from build123d import *

# Parameters (mm, degrees)
SKETCH1_R           = 1.5
SKETCH1_R_2         = 55
BOSS_EXTRUDE1_DEPTH = 3.175
CUT_EXTRUDE3_DEPTH  = 140.736059076
CUT_EXTRUDE4_START  = -10
SKETCH3_R           = 1.5
CUT_EXTRUDE4_DEPTH  = 10
CUT_EXTRUDE5_DEPTH  = 140.736059076
CUT_EXTRUDE6_DEPTH  = 140.736059076
SKETCH6_R           = 1.5
CUT_EXTRUDE7_DEPTH  = 124.953233311
SKETCH7_W           = 69.762043991
SKETCH7_H           = 61.208981149
CUT_EXTRUDE8_DEPTH  = 100


with BuildPart() as part:
    # Sketch1 → Boss-Extrude1 (new body)
    with BuildSketch(Plane(origin=(0, 0, 0), x_dir=(1, 0, 0), z_dir=(0, 1, 0))):
        Polygon((0.047005036, -98.782806148), (-98.782806148, -0.047005036), (-0.047005036, 98.782806148), (98.782806148, 0.047005036), align=None)
        with Locations(Location((-61.346730494, 5.55625, 0), (0, 0, 270))):
            Circle(SKETCH1_R, mode=Mode.SUBTRACT)
        with Locations(Location((-61.346730494, -5.55625, 0), (0, 0, 270))):
            Circle(SKETCH1_R, mode=Mode.SUBTRACT)
        with Locations(Location((-5.55625, -61.346730494, 0), (0, 0, 270))):
            Circle(SKETCH1_R, mode=Mode.SUBTRACT)
        with Locations(Location((5.55625, -61.346730494, 0), (0, 0, 270))):
            Circle(SKETCH1_R, mode=Mode.SUBTRACT)
        with Locations(Location((61.346730494, -5.55625, 0), (0, 0, 270))):
            Circle(SKETCH1_R, mode=Mode.SUBTRACT)
        with Locations(Location((61.346730494, 5.55625, 0), (0, 0, 270))):
            Circle(SKETCH1_R, mode=Mode.SUBTRACT)
        with Locations(Location((5.55625, 61.346730494, 0), (0, 0, 270))):
            Circle(SKETCH1_R, mode=Mode.SUBTRACT)
        with Locations(Location((-5.55625, 61.346730494, 0), (0, 0, 270))):
            Circle(SKETCH1_R, mode=Mode.SUBTRACT)
        with Locations(Location((0, 0, 0), (0, 0, 270))):
            Circle(SKETCH1_R_2, mode=Mode.SUBTRACT)
    extrude(amount=BOSS_EXTRUDE1_DEPTH)

    # Sketch2 → Cut-Extrude3 (cut, through all)
    with BuildSketch(Plane(origin=(0, 3.175, 0), x_dir=(1, 0, 0), z_dir=(0, 1, 0))):
        Polygon((3.175, 53.34), (3.175, 59.69), (-3.175, 59.69), (-3.175, 53.34), (-3.175, 52.244537665), (3.175, 52.244537665), align=None)
        Polygon((53.34, -3.175), (59.69, -3.175), (59.69, 3.175), (53.34, 3.175), (52.244537665, 3.175), (52.244537665, -3.175), align=None)
        Polygon((-3.175, -53.34), (-3.175, -59.69), (3.175, -59.69), (3.175, -53.34), (3.175, -52.244537665), (-3.175, -52.244537665), align=None)
        Polygon((-53.34, 3.175), (-59.69, 3.175), (-59.69, -3.175), (-53.34, -3.175), (-52.244537665, -3.175), (-52.244537665, 3.175), align=None)
    extrude(amount=-CUT_EXTRUDE3_DEPTH, mode=Mode.SUBTRACT)

    # Sketch3 → Cut-Extrude4 (cut)
    # profile 1 of 3: a face of its own
    with BuildSketch(Plane(origin=(0, 3.175, 0), x_dir=(1, 0, 0), z_dir=(0, 1, 0)).offset(CUT_EXTRUDE4_START)):
        with BuildLine():
            Line((38.872362643, 38.909374482), (49.367900556, 49.414905592))
            Line((49.367900556, 49.414905592), (24.66044776, 74.09885587))
            Line((24.66044776, 74.09885587), (5.321919094, 54.741914263))
            ThreePointArc((5.321919094, 54.741914263), (23.472344653, 49.739813394), (38.872362643, 38.909374482))
        make_face()
    # profile 2 of 3: a face of its own
    with BuildSketch(Plane(origin=(0, 3.175, 0), x_dir=(1, 0, 0), z_dir=(0, 1, 0)).offset(CUT_EXTRUDE4_START)):
        with BuildLine():
            Line((-49.367900556, -49.414905592), (-38.872362643, -38.909374482))
            ThreePointArc((-38.872362643, -38.909374482), (-49.717452606, -23.519670626), (-54.736824686, -5.374013707))
            Line((-54.736824686, -5.374013707), (-74.075353352, -24.730955314))
            Line((-74.075353352, -24.730955314), (-49.367900556, -49.414905592))
        make_face()
    # profile 3 of 3: a face of its own
    with BuildSketch(Plane(origin=(0, 3.175, 0), x_dir=(1, 0, 0), z_dir=(0, 1, 0)).offset(CUT_EXTRUDE4_START)):
        with BuildLine():
            Line((98.782806148, 0.047005036), (49.367900556, 49.414905592))
            Line((49.367900556, 49.414905592), (38.872362643, 38.909374482))
            ThreePointArc((38.872362643, 38.909374482), (50.179066182, 22.518022052), (54.908281479, 3.175))
            Line((54.908281479, 3.175), (59.69, 3.175))
            Line((59.69, 3.175), (59.69, -3.175))
            Line((59.69, -3.175), (54.908281479, -3.175))
            ThreePointArc((54.908281479, -3.175), (38.890872965, -38.890872965), (3.175, -54.908281479))
            Line((3.175, -54.908281479), (3.175, -59.69))
            Line((3.175, -59.69), (-3.175, -59.69))
            Line((-3.175, -59.69), (-3.175, -54.908281479))
            ThreePointArc((-3.175, -54.908281479), (-22.494142184, -50.189775527), (-38.872362643, -38.909374482))
            Line((-38.872362643, -38.909374482), (-49.367900556, -49.414905592))
            Line((-49.367900556, -49.414905592), (0.047005036, -98.782806148))
            Line((0.047005036, -98.782806148), (98.782806148, 0.047005036))
        make_face()
        with Locations((-5.55625, -61.346730494)):
            Circle(SKETCH3_R, mode=Mode.SUBTRACT)
        with Locations((5.55625, -61.346730494)):
            Circle(SKETCH3_R, mode=Mode.SUBTRACT)
        with Locations((61.346730494, -5.55625)):
            Circle(SKETCH3_R, mode=Mode.SUBTRACT)
        with Locations((61.346730494, 5.55625)):
            Circle(SKETCH3_R, mode=Mode.SUBTRACT)
    extrude(amount=CUT_EXTRUDE4_DEPTH, mode=Mode.SUBTRACT)

    # Sketch4 → Cut-Extrude5 (cut, through all)
    with BuildSketch(Plane(origin=(0, 3.175, 0), x_dir=(1, 0, 0), z_dir=(0, 1, 0))):
        Polygon((-54.908281479, 3.175), (-75.255419375, 23.502783048), (-23.546766486, 75.260669691), (-3.175, 54.908281479), align=None)
    extrude(amount=-CUT_EXTRUDE5_DEPTH, mode=Mode.SUBTRACT)


with BuildPart() as cut_extrude5_piece_1:
    # of the separate pieces the step leaves, piece 1, a body of its own (cut_extrude5_pieces)
    add(part.part.solids().sort_by_distance((-74.075353352, 0, 24.730955314))[0])


with BuildPart() as cut_extrude5_piece_2:
    # of the separate pieces the step leaves, piece 2, a body of its own (cut_extrude5_pieces)
    add(part.part.solids().sort_by_distance((-3.175, 0, -54.908281479))[0])


with BuildPart() as cut_extrude6_tool:
    # Sketch5 → Cut-Extrude6 (new, through all)
    with BuildSketch(Plane(origin=(0, 3.175, 0), x_dir=(1, 0, 0), z_dir=(0, 1, 0))):
        Polygon((-0.047005036, 98.782806148), (11.121699276, 87.624725864), (-87.614101836, -11.205085321), (-98.782806148, -0.047005036), align=None)
    extrude(amount=-CUT_EXTRUDE6_DEPTH)


with BuildPart() as cut_extrude5_piece_1_1:
    add(cut_extrude5_piece_1.part)

    # Cut-Extrude6: cut by cut_extrude6_tool
    add(cut_extrude6_tool.part, mode=Mode.SUBTRACT)


with BuildPart() as cut_extrude5_piece_2_1:
    add(cut_extrude5_piece_2.part)

    # Cut-Extrude6: cut by cut_extrude6_tool
    add(cut_extrude6_tool.part, mode=Mode.SUBTRACT)


with BuildPart() as cut_extrude7_tool:
    # Sketch6 → Cut-Extrude7 (new, through all)
    with BuildSketch(Plane(origin=(0, 3.175, 0), x_dir=(1, 0, 0), z_dir=(0, 1, 0))):
        with BuildLine():
            ThreePointArc((-73.220428508, -14.983508678), (-73.219419094, -17.104828781), (-71.09809899, -17.103819368))
            Line((-71.09809899, -17.103819368), (-73.220428508, -14.983508678))
        make_face()
        with BuildLine():
            Line((-73.220428508, -14.983508678), (-71.09809899, -17.103819368))
            ThreePointArc((-71.09809899, -17.103819368), (-70.773307917, -16.617359439), (-70.659263749, -16.043664023))
            ThreePointArc((-70.659263749, -16.043664023), (-71.585568332, -14.657708191), (-73.220428508, -14.983508678))
        make_face()
        with BuildLine():
            ThreePointArc((-79.989802749, -8.220573681), (-79.988793336, -10.341893785), (-77.867473232, -10.340884371))
            Line((-77.867473232, -10.340884371), (-79.989802749, -8.220573681))
        make_face()
        with BuildLine():
            Line((-79.989802749, -8.220573681), (-77.867473232, -10.340884371))
            ThreePointArc((-77.867473232, -10.340884371), (-77.542682159, -9.854424443), (-77.428637991, -9.280729026))
            ThreePointArc((-77.428637991, -9.280729026), (-78.354942574, -7.894773194), (-79.989802749, -8.220573681))
        make_face()
        with Locations(Location((16.002609239, 72.202151202, 0), (0, 0, 270))):
            Circle(SKETCH6_R)
        with Locations(Location((9.233234997, 78.965086199, 0), (0, 0, 270))):
            Circle(SKETCH6_R)
    extrude(amount=-CUT_EXTRUDE7_DEPTH)


with BuildPart() as cut_extrude5_piece_1_2:
    add(cut_extrude5_piece_1_1.part)

    # Cut-Extrude7: cut by cut_extrude7_tool
    add(cut_extrude7_tool.part, mode=Mode.SUBTRACT)

    # Sketch7 → Cut-Extrude8 (cut)
    with BuildSketch(Plane(origin=(-49.367900556, 0, 49.414905592), x_dir=(0.7074431724013648, 0, 0.7067702298644821), z_dir=(-0.7067702298644821, 0, 0.7074431724013648))):
        with Locations((-46.400178309, 4.239305035)):
            Rectangle(SKETCH7_W, SKETCH7_H)
    extrude(amount=-CUT_EXTRUDE8_DEPTH, mode=Mode.SUBTRACT)


with BuildPart() as cut_extrude5_piece_2_2:
    add(cut_extrude5_piece_2_1.part)

    # Cut-Extrude7: cut by cut_extrude7_tool
    add(cut_extrude7_tool.part, mode=Mode.SUBTRACT)


solid = cut_extrude5_piece_2_2.part
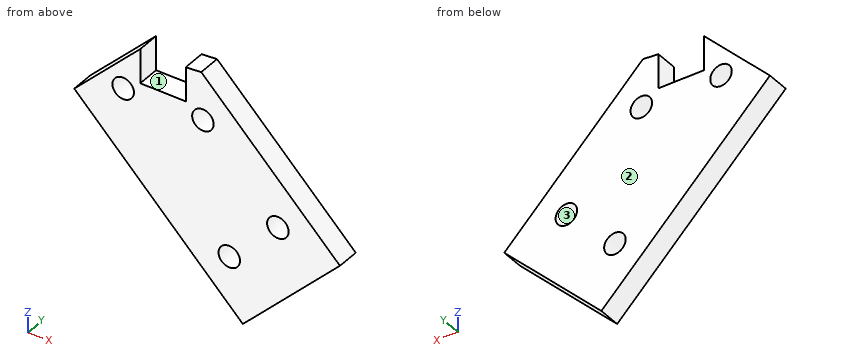
For this review, take the finished solid that the model builds, in its own axes (mm). Face numbers are marked on the shaded views. Give positions to 0.01 mm unless a question says otherwise; leave off trailing zeros. Loops run counter-clockwise (first coordinate to the right, second up) from the corner with the lowest first, then second, coordinate; pieces in that order, holes last.
Item 1: Take a section at C-C, the plane y = 1.8. State the section outline as (x, z) points (3 decimals), and give its area (3 significant figures).
Item 2: For line 1 along X through (y, z) = (2.4, -73.5); line 2 along X through (y, z) = (2.5, -78); line 3 along Z through (x, y) = (-2.5, 2.85), list the stretches that pass through material, from the lowest coordinate up.
Item 3: Take a section at D-D, the plane x = 0.5. State the section outline as (y, z) points (3 decimals), and give its area (3 significant figures).
Item 4: Insertion check: pin 1 (1.6 mm diameter, centred on x = 1, y = 1, fed in from +Z); pin 2 (1.6 mm diameter, centred on y = 2, z = -57, fed in from -X); pin 3 (12 mm diameter, centred on x = 14.5, z = -60, fed in from -Y); pin 4 (1 mm diameter, centred on y = 1.5, z = -57.5, fed in from +X). Each pin has a flat end and moves straight along its axis. Give the tip position at first contact, or say it passes through.
Item 5: Take a section at B-B, the plane x = 8.5. State the section outline as (y, z) points (3 decimals), and give its area (3 significant figures).
Item 6: Take a section at A-A, the plane z = -79. State the section outline as (x, y) points (3 decimals).
Item 7: Draft analysis for pull direction Z (two halves, no side actions). For the marked faces 1, 2 and 3, state which applies: +Z half, -Z half, draft (parallel to the pull), parting line (faces both ways), or undercut.
Calculated:
1. outline: (-12.378, -64.103) - (11.122, -87.625) - (24.66, -74.099) - (5.322, -54.742) arc R55 cw to (3.175, -54.908) - (3.175, -59.69) - (-3.175, -59.69) - (-3.175, -54.908) - close; hole circle Ø3 at (-5.556, -61.347); hole circle Ø3 at (5.556, -61.347); hole circle Ø3 at (9.233, -78.965); hole circle Ø3 at (16.003, -72.202)
1. area: 559 mm2
2. line 1: x = -2.99 to 15.25, 16.75 to 24.06
2. line 2: x = 1.51 to 8.08, 10.38 to 20.76
2. line 3: z = -73.99 to -59.69
3. outline: (0, -76.993) - (3.175, -76.993) - (3.175, -59.69) - (0, -59.69) - close
3. area: 54.9 mm2
4. pin 1: stops at z = -59.69
4. pin 2: stops at x = -6.07
4. pin 3: stops at y = 0
4. pin 4: stops at x = 8.58
5. outline: (0, -85.001) - (3.175, -85.001) - (3.175, -80.274) - (0, -80.274) - close; (0, -77.657) - (3.175, -77.657) - (3.175, -57.923) - (0, -57.923) - close
5. area: 77.7 mm2
6. outline: (2.505, 0) - (7.734, 0) - (7.734, 3.175) - (2.505, 3.175) - close; (10.733, 0) - (19.755, 0) - (19.755, 3.175) - (10.733, 3.175) - close
7. face 1: +Z half
7. face 2: draft
7. face 3: undercut
